Geometry check sheet. Reference: the model listing, model coordinates, mm. Face numbers are marked on the shaded views. A direction names the side the tool comes from. Round coordinates to 2 decimals unless told otherwise and drop trailing zeros. Loops run counter-clockwise (first coordinate to the right, second up) from the corner with the lowest first, then second, coordinate; pieces in that order, holes last. Notation, with made-up numbers: M 73.25,45 L 114.25,45 A18 cw 114.25,80 Z; hole C 16,-9 d2. An arc over 180 degrees is marked long. Write item = value, one per line.
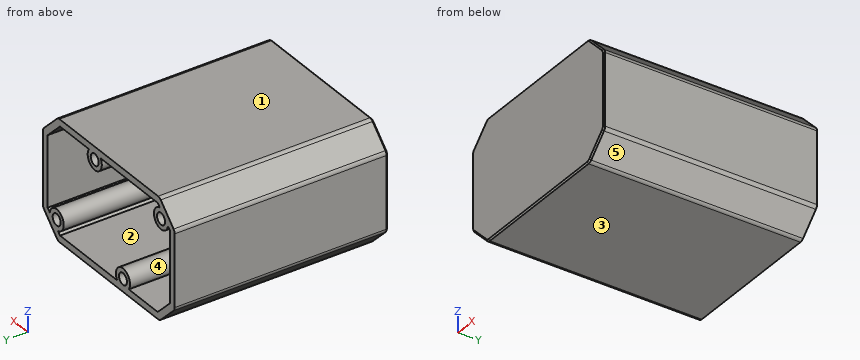
from build123d import *

# Parameters (mm, degrees)
BOSS_EXTRUDE1_DEPTH = 3
SKETCH1_4_R         = 2.125
BOSS_EXTRUDE2_DEPTH = 78
CHAMFER1_SIZE       = 0.5


with BuildPart() as part:
    # Sketch1 → Boss-Extrude1 (new body)
    with BuildSketch(Plane(origin=(0, 0, 0), x_dir=(1, 0, 0), z_dir=(0, 1, 0))):
        with BuildLine():
            Line((26.171572875, 22), (-26.171572875, 22))
            ThreePointArc((-26.171572875, 22), (-26.93693974, 21.847759065), (-27.585786438, 21.414213562))
            Line((-27.585786438, 21.414213562), (-34.414213562, 14.585786438))
            ThreePointArc((-34.414213562, 14.585786438), (-34.847759065, 13.93693974), (-35, 13.171572875))
            Line((-35, 13.171572875), (-35, -13.171572875))
            ThreePointArc((-35, -13.171572875), (-34.847759065, -13.93693974), (-34.414213562, -14.585786438))
            Line((-34.414213562, -14.585786438), (-27.585786438, -21.414213562))
            ThreePointArc((-27.585786438, -21.414213562), (-26.93693974, -21.847759065), (-26.171572875, -22))
            Line((-26.171572875, -22), (26.171572875, -22))
            ThreePointArc((26.171572875, -22), (26.93693974, -21.847759065), (27.585786438, -21.414213562))
            Line((27.585786438, -21.414213562), (34.414213562, -14.585786438))
            ThreePointArc((34.414213562, -14.585786438), (34.847759065, -13.93693974), (35, -13.171572875))
            Line((35, -13.171572875), (35, 13.171572875))
            ThreePointArc((35, 13.171572875), (34.847759065, 13.93693974), (34.414213562, 14.585786438))
            Line((34.414213562, 14.585786438), (27.585786438, 21.414213562))
            ThreePointArc((27.585786438, 21.414213562), (26.93693974, 21.847759065), (26.171572875, 22))
        make_face()
    extrude(amount=BOSS_EXTRUDE1_DEPTH)

    # Sketch1<4> → Boss-Extrude2 (add)
    with BuildSketch(Plane(origin=(0, 0, 0), x_dir=(1, 0, 0), z_dir=(0, 1, 0))):
        with BuildLine():
            ThreePointArc((27.585786438, 21.414213562), (26.93693974, 21.847759065), (26.171572875, 22))
            Line((26.171572875, 22), (-26.171572875, 22))
            ThreePointArc((-26.171572875, 22), (-26.93693974, 21.847759065), (-27.585786438, 21.414213562))
            Line((-27.585786438, 21.414213562), (-34.414213562, 14.585786438))
            ThreePointArc((-34.414213562, 14.585786438), (-34.847759065, 13.93693974), (-35, 13.171572875))
            Line((-35, 13.171572875), (-35, -13.171572875))
            ThreePointArc((-35, -13.171572875), (-34.847759065, -13.93693974), (-34.414213562, -14.585786438))
            Line((-34.414213562, -14.585786438), (-27.585786438, -21.414213562))
            ThreePointArc((-27.585786438, -21.414213562), (-26.93693974, -21.847759065), (-26.171572875, -22))
            Line((-26.171572875, -22), (26.171572875, -22))
            ThreePointArc((26.171572875, -22), (26.93693974, -21.847759065), (27.585786438, -21.414213562))
            Line((27.585786438, -21.414213562), (34.414213562, -14.585786438))
            ThreePointArc((34.414213562, -14.585786438), (34.847759065, -13.93693974), (35, -13.171572875))
            Line((35, -13.171572875), (35, 13.171572875))
            ThreePointArc((35, 13.171572875), (34.847759065, 13.93693974), (34.414213562, 14.585786438))
            Line((34.414213562, 14.585786438), (27.585786438, 21.414213562))
        make_face()
        with BuildLine():
            Line((-32.5, -12.964466094), (-32.5, 12.964466094))
            Line((-32.5, 12.964466094), (-25.964466094, 19.5))
            Line((-25.964466094, 19.5), (-10.589801774, 19.5))
            ThreePointArc((-10.589801774, 19.5), (-7.5, 13.625), (-4.410198226, 19.5))
            Line((-4.410198226, 19.5), (25.964466094, 19.5))
            Line((25.964466094, 19.5), (27.04741326, 18.417052834))
            ThreePointArc((27.04741326, 18.417052834), (25.077980708, 12.077980708), (31.417052834, 14.04741326))
            Line((31.417052834, 14.04741326), (32.5, 12.964466094))
            Line((32.5, 12.964466094), (32.5, -12.964466094))
            Line((32.5, -12.964466094), (25.964466094, -19.5))
            Line((25.964466094, -19.5), (10.589801774, -19.5))
            ThreePointArc((10.589801774, -19.5), (7.5, -13.625), (4.410198226, -19.5))
            Line((4.410198226, -19.5), (-25.964466094, -19.5))
            Line((-25.964466094, -19.5), (-27.04741326, -18.417052834))
            ThreePointArc((-27.04741326, -18.417052834), (-25.077980708, -12.077980708), (-31.417052834, -14.04741326))
            Line((-31.417052834, -14.04741326), (-32.5, -12.964466094))
        make_face(mode=Mode.SUBTRACT)
        with Locations(Location((-27.729631137, -14.729631137, 0), (0, 0, 270))):
            Circle(SKETCH1_4_R, mode=Mode.SUBTRACT)
        with Locations(Location((-7.5, 17.375, 0), (0, 0, 270))):
            Circle(SKETCH1_4_R, mode=Mode.SUBTRACT)
        with Locations(Location((7.5, -17.375, 0), (0, 0, 270))):
            Circle(SKETCH1_4_R, mode=Mode.SUBTRACT)
        with Locations(Location((27.729631137, 14.729631137, 0), (0, 0, 270))):
            Circle(SKETCH1_4_R, mode=Mode.SUBTRACT)
    extrude(amount=BOSS_EXTRUDE2_DEPTH)

    # Chamfer1
    chamfer1_edges = [part.edges().sort_by_distance(p)[0] for p in [
        (-31, 0, 18),
        (-34.847759065, 0, 13.93693974),
        (-35, 0, 0),
        (-34.847759065, 0, -13.93693974),
        (-31, 0, -18),
        (-26.93693974, 0, -21.847759065),
        (0, 0, -22),
        (26.93693974, 0, -21.847759065),
        (31, 0, -18),
        (34.847759065, 0, -13.93693974),
        (35, 0, 0),
        (34.847759065, 0, 13.93693974),
        (31, 0, 18),
        (26.93693974, 0, 21.847759065),
        (0, 0, 22),
        (-26.93693974, 0, 21.847759065),
    ]]
    chamfer(chamfer1_edges, length=CHAMFER1_SIZE)


solid = part.part
(1) Tool access check on the marked faces 1 and 2. Record the directions out of +Z, -Z, +X, -X, +Y, -Y that give a thin tool (end or side, any length) a straight path to the whole face; none if there is none.
Result set:
face_1 = +Z, +X, -X, +Y, -Y
face_2 = +Y
(2) Release check for a two-part mould opening along X. For the marked faces 3, 4 and 5 record: released by +X, released by -X, zero draft, split by the parting line, or undercut.
Result set:
face_3 = zero draft
face_4 = undercut
face_5 = released by +X
(3) Sectioned sample at B-B on x = 22. Record the cut outline in (y, z), then the cut area to 3 significant figures.
Result set:
outline = M 0,-21.5 L 0.5,-22 L 78,-22 L 78,-19.5 L 3,-19.5 L 3,19.5 L 78,19.5 L 78,22 L 0.5,22 L 0,21.5 Z
area = 507 mm2
(4) Sectioned sample at D-D on y = 67. State how many separate pieces and enclosed holes the cut face has, then the cut area to 4 significant figures.
Result set:
separate_pieces = 1
enclosed_holes = 5
area = 593.5 mm2
(5) Sectioned sample at C-C on x = -7.5. Record the cut outline in (y, z) (3 decimals), then the cut area to 3 significant figures.
Result set:
outline = M 0,-21.5 L 0.5,-22 L 78,-22 L 78,-19.5 L 3,-19.5 L 3,-15.25 L 78,-15.25 L 78,-13.625 L 3,-13.625 L 3,19.5 L 78,19.5 L 78,22 L 0.5,22 L 0,21.5 Z
area = 629 mm2
(6) Depth check by flat-ended pin: pin 1 Ø11.5 at (x, z) = (7, 1.5) entering from +Y; pin 2 Ø3 at (y, z) = (22.5, 16) entering from -X. Enter the tip coordinate at first touch or a pass-through.
Result set:
pin_1 = 3
pin_2 = -34.5
(7) Sectioned sample at A-A on z = -1. Record the cut outline in (x, y).
Result set:
outline = M -35,0.5 L -34.5,0 L 34.5,0 L 35,0.5 L 35,78 L 32.5,78 L 32.5,3 L -32.5,3 L -32.5,78 L -35,78 Z
(8) Material ranges on line 1 along Z through (x, y) = (7.5, 58.5) (3 decimals); line 2 along X through (y, z) = (35.5, -10); line 3 along Z through (x, y) = (-18, 33.5), recorded low to high. Write a range as from..to.
Result set:
line_1 = -22..-19.5, 13.625..15.25, 19.5..22
line_2 = -35..-32.5, 32.5..35
line_3 = -22..-19.5, 19.5..22
